```python
from build123d import *

# Parameters (mm, degrees)
SKETCH_1_W      = 40
SKETCH_1_H      = 20
EXTRUDE_1_DEPTH = 39.5
SKETCH_2_R      = 3
SKETCH_2_R_2    = 1.5
EXTRUDE_2_DEPTH = 3.5
SKETCH_4_W      = 56
SKETCH_4_H      = 20
SKETCH_4_R      = 2
EXTRUDE_3_DEPTH = 2.5


with BuildPart() as part:
    # 草图1 → 凸台-拉伸1 (new body)
    with BuildSketch(Plane.XY):
        Rectangle(SKETCH_1_W, SKETCH_1_H)
    extrude(amount=EXTRUDE_1_DEPTH)

    # 草图2 → 凸台-拉伸2 (add)
    with BuildSketch(Plane.XY.offset(39.5)):
        with Locations(Location((10, 0, 0), (0, 0, 180))):
            Circle(SKETCH_2_R)
        with Locations((10, 0)):
            Circle(SKETCH_2_R_2, mode=Mode.SUBTRACT)
    extrude(amount=EXTRUDE_2_DEPTH)

    # 草图4 → 凸台-拉伸3 (add)
    with BuildSketch(Plane.XY.offset(33.5)):
        Rectangle(SKETCH_4_W, SKETCH_4_H)
        with Locations((25, 5)):
            Circle(SKETCH_4_R, mode=Mode.SUBTRACT)
        with Locations((25, -5)):
            Circle(SKETCH_4_R, mode=Mode.SUBTRACT)
        with Locations((-25, 5)):
            Circle(SKETCH_4_R, mode=Mode.SUBTRACT)
        with Locations((-25, -5)):
            Circle(SKETCH_4_R, mode=Mode.SUBTRACT)
    extrude(amount=-EXTRUDE_3_DEPTH)


solid = part.part
```
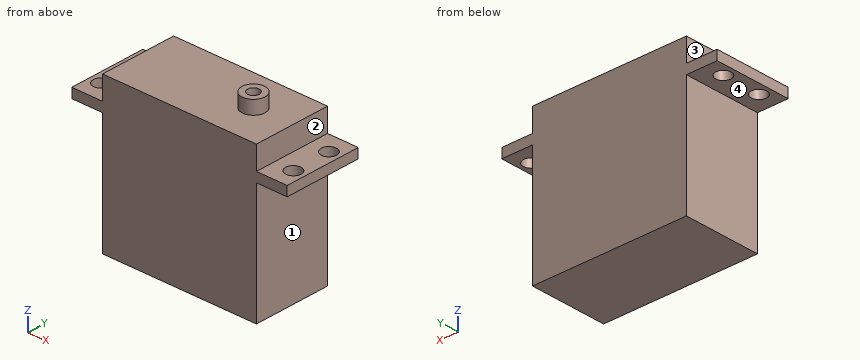
Design review of the part built by this model. Coordinates are the model's own, in mm. Face numbers are marked on the shaded views. A direction names the side the tool comes from. Coordinates: 2 decimals unless noted, no trailing zeros. Order: outer loops, then holes, each group sorted by start corner. A loop starts at its lowest first (then second) coordinate and runs counter-clockwise, first axis right, second up. Notation, with made-up numbers: M -35,32 L 10,32 A18 ccw 10,52 Z; hole C -31,-31.5 d5. An arc over 180 degrees is marked long. Answer as a JSON object with one key per item and string values. Group by question number.
1) Add section B-B, the plane x = -25. Write out the cut boundary in (y, z).
2) Add section D-D, the plane z = 37. Write out the cut boundary in (x, y).
3) Add section A-A, the plane y = -5. Write out the cut boundary in (x, z).
4) For pin 1 (1.8 mm diameter, centred on y = -1, z = 37.5, fed in from -X); pin 2 (9 mm diameter, centred on x = 26, y = -1, fed in from +Z); pin 3 (6 mm diameter, centred on x = -9.5, y = -4.5, fed in from +Z), all flat-tipped, find the tip position at first contact; note any pin that passes through.
5) Tool access review of the marked faces 1, 2, 3 and 4: name each direction out of +Z, -Z, +X, -X, +Y, -Y from which nothing blocks a thin tool from reaching the whole face with its end or side.
6) Add section C-C, the plane x = 10. Write out the cut boundary in (y, z), then the cut area to 4 significant figures.
7) Wall thickness on L1, parallel to Y at x = 25, z = 33; L2, parallel to Z at x = 7.5, y = 7.75; L3, parallel to Y at x = 10, z = 41.45: over which ranges is each line inside the solid? List them lowest first.
Computed values:
{
 "1": {"outline": "M -10,31 L -7,31 L -7,33.5 L -10,33.5 Z; M -3,31 L 3,31 L 3,33.5 L -3,33.5 Z; M 7,31 L 10,31 L 10,33.5 L 7,33.5 Z"},
 "2": {"outline": "M -20,-10 L 20,-10 L 20,10 L -20,10 Z"},
 "3": {"outline": "M -28,31 L -27,31 L -27,33.5 L -28,33.5 Z; M -23,31 L -20,31 L -20,0 L 20,0 L 20,31 L 23,31 L 23,33.5 L 20,33.5 L 20,39.5 L -20,39.5 L -20,33.5 L -23,33.5 Z; M 27,31 L 28,31 L 28,33.5 L 27,33.5 Z"},
 "4": {"pin 1": "stops at x = -20", "pin 2": "stops at z = 33.5", "pin 3": "stops at z = 39.5"},
 "5": {"face 1": "-Z, +X, +Y, -Y", "face 2": "+Z, +X, +Y, -Y", "face 3": "+Z, -X, +Y, -Y", "face 4": "-Z, -X, +Y, -Y"},
 "6": {"outline": "M -10,0 L 10,0 L 10,39.5 L 3,39.5 L 3,43 L 1.5,43 L 1.5,39.5 L -1.5,39.5 L -1.5,43 L -3,43 L -3,39.5 L -10,39.5 Z", "area": "800.5 mm^2"},
 "7": {"L1": "y = -10 to -7, -3 to 3, 7 to 10", "L2": "z = 0 to 39.5", "L3": "y = -3 to -1.5, 1.5 to 3"}
}
